Design review of the part built by this model. Coordinates are the model's own, in mm. Give positions to 0.01 mm unless a question says otherwise; leave off trailing zeros. Use CSV: the item, a comma, the result in double quotes.
Autodesk Inventor part; units mm, degrees
ref_plane "YZ Plane" through (0, 0, 0) normal (1, 0, 0) x (0, 1, 0)
ref_plane "XZ Plane" through (0, 0, 0) normal (0, 1, 0) x (-1, 0, 0)
ref_plane "XY Plane" through (0, 0, 0) normal (0, 0, 1) x (1, 0, 0)
sketch "スケッチ1" plane through (0, 0, 0) normal (1, 0, 0) x (0, 1, 0)
  line L0 (27, 0) -> (0, 0)
  line L1 (0, 0) -> (0, -65.8723)
  line L2 (0, -65.8723) -> (27, -65.8723)
  line L3 (27, -65.8723) -> (27, 0)
  line L4 (0, 0) -> (19.7037, 34.1277)
  line L5 (19.7037, 34.1277) -> (43.0863, 20.6277)
  line L6 (43.0863, 20.6277) -> (27, -7.2346)
  line L7 (27, 19.7654) -> (31.395, 27.3777)
  circle A0 centre (27, 19.7654) radius 6.25
  circle A1 centre (13.5, -57.0823) radius 6.25
  line L8 (13.5, -65.8723) -> (13.5, -57.0823)
  circle A2 centre (27, 19.7654) radius 13.5
  circle A3 centre (13.5, -57.0823) radius 13.5
  circle A4 centre (13.5, -57.0823) radius 13
  line L9 (37, -44.0823) -> (13.5, -44.0823)
  line L10 (13.5, -44.0823) -> (13.5, -70.0823)
  line L11 (13.5, -70.0823) -> (37, -70.0823)
  line L12 (37, -70.0823) -> (37, -44.0823)
  line L13 (8, 13.8564) -> (8, -44.7534)
  line L14 (8, -44.7534) -> (8, -45.303)
  point P0 (38.6913, 13.0154)
  point P1 (15.3087, 26.5154)
  point P2 (0, -57.0823)
  point P3 (27, -57.0823)
  point P4 (0, -57.0823)
  point P5 (27, -44.0823)
  point P6 (40.2685, 22.2546)
  point P7 (22.5215, 32.5009)
  point P8 (8, 0)
  point P9 (17.1401, -44.0823)
  point P10 (13.5, -44.0823)
  dimension "d23" = 26
  dimension "d0" = 27
  dimension "d4" = 150
  dimension "d5" = 90
  dimension "d6" = 27
  dimension "d12" = 8.79
  dimension "d13" = 8.79
  dimension "d14" = 12.5
  dimension "d17" = 100
  dimension "d24" = 23.5
  dimension "d30" = 8
extrude "押し出し1" add sketch "スケッチ1" along normal blind 1.5 contours L3 L9 A3 L13 L0 | L0 L13 L4 A2 L6 L3 | L0 L4 L13 | A3 L9 A4 L14 | L9 L12 L11 A3 L2 L3 | L3 A3 L9 | A0 | A2 L5 | A3 L2 A4 L9 | A4 L10 A1 L8 L2 | L3 L2 A3 | A2 L5 | A4 L2 L8 A1 L10 | L2 L10 A4 | A3 L11 A4 L2 | L10 L8 A1 | A1 L8 L10 | L2 A4 L10 picked at (17.348, -69.6234)
extrude "押し出し2" cut sketch "スケッチ1" along normal blind 1.5 contours A0 | L10 L8 A1 | A1 L8 L10
fillet "フィレット1" radius 8 5 edges at (0.75, 27, -7.2346) (0.75, 27, -44.0823) (0.75, 8, -45.303) (0.75, 8, 0) (0.75, 0, 0)
fillet "フィレット2" radius 3 2 edges at (0.75, 37, -70.0823) (0.75, 37, -44.0823)
sketch "スケッチ6" plane through (1.5, 0, 0) normal (1, 0, 0) x (0, 0, -1)
  circle A0 centre (67.5823, 34.5) radius 0.85
  circle A1 centre (46.5823, 34.5) radius 0.85
  circle A2 centre (67.5823, 13.5) radius 0.85
  circle A3 centre (46.5823, 13.5) radius 0.85
  circle A4 centre (-6.8288, 7.4067) radius 0.85
  circle A5 centre (-25.0154, 17.9067) radius 0.85
  circle A6 centre (-14.5154, 36.0933) radius 0.85
  circle A7 centre (3.6712, 25.5933) radius 0.85
  line L0 (35.8933, 18.515) -> (30.098, 15.8126)
  line L1 (30.9432, 12) -> (35.3442, 12)
  line L2 (36.1894, 12.1874) -> (37.5838, 12.8376)
  line L3 (38.7385, 14.6502) -> (38.7385, 16.7024)
  line L4 (27.0251, 23) -> (11.2026, 23)
  line L5 (9.4706, 22) -> (5.4291, 15)
  line L6 (7.1612, 12) -> (12.0136, 12)
  line L7 (12.8588, 12.1874) -> (27.8704, 19.1874)
  line L8 (42.7385, 10.8278) -> (36.6744, 8)
  line L9 (3.1834, 8) -> (36.6744, 8)
  arc A8 (2.1834, 8.2679) -> (3.1834, 8) centre (3.1834, 10) ccw
  line L10 (-0.0294, 9.5455) -> (2.1834, 8.2679)
  arc A9 (-0.7615, 12.2776) -> (-0.0294, 9.5455) centre (0.9706, 11.2776) ccw
  line L11 (7.1612, 26) -> (-0.7615, 12.2776)
  arc A10 (8.8932, 27) -> (7.1612, 26) centre (8.8932, 25) ccw
  line L12 (40.7385, 27) -> (8.8932, 27)
  line L13 (42.7385, 10.8278) -> (42.7385, 25)
  circle A11 centre (-19.7654, 27) radius 6.25
  circle A12 centre (57.0823, 13.5) radius 6.25
  line L14 (-14.5154, 36.0933) -> (3.6712, 25.5933)
  line L15 (3.6712, 25.5933) -> (-6.8288, 7.4067)
  line L16 (-6.8288, 7.4067) -> (-25.0154, 17.9067)
  line L17 (-25.0154, 17.9067) -> (-14.5154, 36.0933)
  line L18 (5.3782, 28.0718) -> (-13.0154, 38.6913)
  line L19 (46.5823, 34.5) -> (67.5823, 34.5)
  line L20 (67.5823, 34.5) -> (67.5823, 13.5)
  line L21 (67.5823, 13.5) -> (46.5823, 13.5)
  line L22 (46.5823, 13.5) -> (46.5823, 34.5)
  line L23 (-16.0154, 33.4952) -> (4.6125, 21.5857)
  line L24 (4.6125, 21.5857) -> (-2.8875, 8.5953)
  line L25 (-2.8875, 8.5953) -> (-23.5154, 20.5048)
  line L26 (-23.5154, 20.5048) -> (-16.0154, 33.4952)
  line L27 (-2.8875, 8.5953) -> (3.1834, 8)
  circle A13 centre (-19.7654, 27) radius 10.25
  circle A14 centre (57.0823, 13.5) radius 10.25
  line L28 (49.5823, 34.5) -> (64.5823, 34.5)
  line L29 (64.5823, 34.5) -> (64.5823, 13.5)
  line L30 (64.5823, 13.5) -> (49.5823, 13.5)
  line L31 (49.5823, 13.5) -> (49.5823, 34.5)
  circle A15 centre (36.0823, 35) radius 12
  arc A16 (36.0823, 27) -> (44.0491, 34.2727) centre (36.0823, 35) ccw
  line L32 (38.7385, 13.376) -> (52.582, 19.8314)
  line L33 (46.5823, 29.1905) -> (49.5823, 34.5)
  arc A17 (35.3442, 12) -> (36.1894, 12.1874) centre (35.3442, 14) ccw
  arc A18 (37.5838, 12.8376) -> (38.7385, 14.6502) centre (36.7385, 14.6502) ccw
  arc A19 (27.8704, 19.1874) -> (27.0251, 23) centre (27.0251, 21) ccw
  arc A20 (11.2026, 23) -> (9.4706, 22) centre (11.2026, 21) ccw
  arc A21 (5.4291, 15) -> (7.1612, 12) centre (7.1612, 14) ccw
  arc A22 (12.0136, 12) -> (12.8588, 12.1874) centre (12.0136, 14) ccw
  arc A23 (30.098, 15.8126) -> (30.9432, 12) centre (30.9432, 14) ccw
  arc A24 (38.7385, 16.7024) -> (35.8933, 18.515) centre (36.7385, 16.7024) ccw
  circle A25 centre (8.8932, 25) radius 0.8
  circle A26 centre (17.4111, 11) radius 0.8
  circle A27 centre (28.9842, 17.5) radius 0.8
  circle A28 centre (0.9706, 11.2776) radius 0.8
  circle A29 centre (40.7385, 25) radius 0.8
  arc A30 (42.7385, 25) -> (40.7385, 27) centre (40.7385, 25) ccw
  point P0 (0, 0)
  point P1 (8, 8)
  point P2 (-7.4164, 4.2819)
  point P3 (42.7385, 15.2413)
  point P4 (47.6605, 17.5364)
  point P5 (64.5823, 20.4866)
  point P6 (48.0718, 34.5)
  point P7 (42.7385, 25.0153)
  point P8 (-17.4648, 17.0115)
  point P9 (-0.7615, 12.2776)
  point P10 (-9.9648, 30.0019)
  point P11 (67.3323, 13.5)
  point P12 (42.7385, 25.0153)
  point P13 (27.138, 27)
  point P14 (46.5823, 17.0336)
  point P15 (46.8323, 13.5)
  point P16 (46.5823, 14.35)
  point P17 (47.4323, 13.5)
  point P18 (67.5823, 14.35)
  point P19 (66.7323, 13.5)
  point P20 (46.5823, 33.65)
  point P21 (47.4323, 34.5)
  point P22 (67.5823, 33.65)
  point P23 (66.7323, 34.5)
  dimension "d31" = 3
  dimension "d32" = 3
  dimension "d33" = 4
  dimension "d34" = 4
  dimension "d35" = 3
  dimension "d36" = 3
  dimension "d37" = 4
extrude "押し出し6" cut sketch "スケッチ6" against normal through all contours A0 L20 L19 | L19 L20 A0 | L29 A14 L31 L19 | L20 L21 A14 A2 | A2 A14 L21 L20 | L31 A14 L32 L22 L33 | A14 L21 A2 | L22 L32 L13 A30 A15 | A2 L21 A14 | L19 L22 A1 | A1 L22 L19 | A14 L21 A3 | A3 L22 L21 A14 | A14 L21 L22 A3 | A3 L21 A14 | L11 L24 L25 L15 L23 | L15 L25 A13 L23 | L15 L14 A7 | A7 L14 L15 | L15 L16 A4 | A4 L16 L15 | A13 L17 L14 A6 | A6 L17 A13 | L14 L17 A13 A6 | A13 L17 A5 | A5 L16 L17 A13 | A6 A13 L17 | A5 A13 L17 L16 | L17 A13 A5 | A24 L3 A18 L2 A17 L1 A23 L0 | A19 L7 A22 L6 A21 L5 A20 L4 | A25 | A26 | A27 | A28 | A29
fillet "フィレット3" radius 2 10 edges at (0.75, 17.0115, 17.4648) (0.75, 30.0019, 9.9648) (0.75, 21.5857, -4.6125) (0.75, 8.5953, 2.8875) (0.75, 15.2413, -42.7385) (0.75, 17.5364, -47.6605) (0.75, 34.5, -49.5823) (0.75, 34.5, -64.5823) (0.75, 20.4866, -64.5823) (0.75, 25.0153, -42.7385)
properties part number "leg_under" material "アルミニウム 6061"
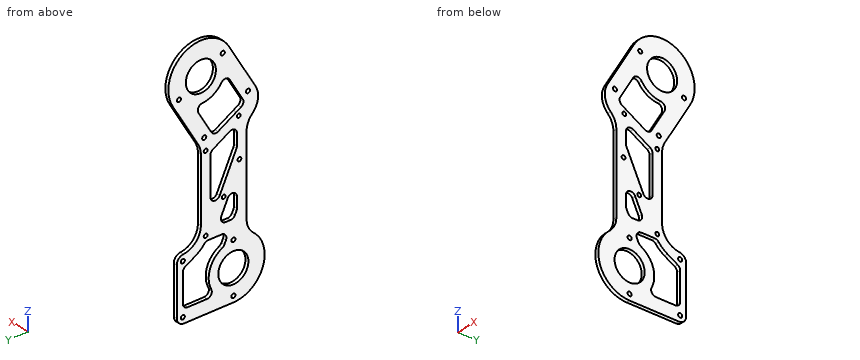
(1) Wall thickness on line 1 along Y through (x, z) = (0.6, -22.5); line 2 along Z through (x, y) = (1.05, 29); line 3 along Y through (x, z) = (1.2, 24.5): over which ranges is each line inside the solid? List them lowest first. Write a range as [from, to].
A:
line 1,"[8, 16.68], [23, 27]"
line 2,"[-70.08, -64.58], [-46.47, -41.37], [-3.77, 13.84], [25.69, 33.12]"
line 3,"[14.15, 17.23], [18.58, 22.92], [31.08, 39.64]"
(2) Clearance check with flat-ended pins moving along their axes: P1, Ø5, axis at y = 22, z = 8.5, coming from the +X side; P2, Ø0.8, axis at x = 1, y = 16, coming from the +Z side; P3, Ø1, axis at y = 25.59, z = -3.67, coming from the +X side. State where each tip first meets the part, or that it passes through.
A:
P1,"x = 1.5"
P2,"z = 28.13"
P3,"through"
(3) We need section A-A on x = 0.75. Count the separate pieces of the cut face and the enclosed holes in it, then the cut area to 3 significant figures.
A:
separate pieces,"1"
enclosed holes,"19"
area,"1,690 mm²"
